Part model, mm, in its own coordinate system. Give positions to 0.01 mm unless a question says otherwise; leave off trailing zeros. Write each loop counter-clockwise with the first axis right and the second up, starting at its lowest first coordinate (ties: lowest second). Pieces come first, ordered by that corner, then holes.
from build123d import *

# Parameters (mm, degrees)
F1_DEPTH = 9.525


with BuildPart() as f1:
    # F0 (on Right) → F1 (new body)
    with BuildSketch(Plane.YZ):
        with BuildLine():
            Line((-686.6, 0), (-54.565425, 0))
            ThreePointArc((-54.565425, 0), (-17.701558, 16.22049), (-4.75569, 54.357787))
            Line((-4.75569, 54.357787), (-56.006549, 640.157787))
            ThreePointArc((-56.006549, 640.157787), (-72.036774, 672.663867), (-105.816284, 685.8))
            Line((-105.816284, 685.8), (-292.97298, 685.8))
            ThreePointArc((-292.97298, 685.8), (-312.355559, 681.890298), (-328.706935, 670.772624))
            Line((-328.706935, 670.772624), (-722.333955, 268.576607))
            ThreePointArc((-722.333955, 268.576607), (-732.896316, 252.489192), (-736.6, 233.603983))
            Line((-736.6, 233.603983), (-736.6, 50))
            ThreePointArc((-736.6, 50), (-721.955339, 14.644661), (-686.6, 0))
        make_face()
    extrude(amount=F1_DEPTH)


solid = f1.part
1) Mould opens along X. For faces 1 (the flat face through (9.525, -294, 272)), 2 (the cylindrical face through (4.696, -722.342, 15.036)), 3 (the flat face through (0, -294, 272)) say: +X half, -X half, draft (parallel to the pull), parting line (faces both ways), or undercut.
Check result:
face 1: +X half
face 2: draft
face 3: -X half
2) Saw through at C-C (z = 524). Write the cut outline in (x, y) (1 decimal).
Check result:
outline: (0, -472.4) - (9.5, -472.4) - (9.5, -45.8) - (0, -45.8) - close
3) Saw through at B-B (y = -474). Write the cut outline in (x, z) (3 decimals).
Check result:
outline: (0, 0) - (9.525, 0) - (9.525, 522.317) - (0, 522.317) - close
4) Drill centre lines: L1, parallel to Z at x = 5.5, y = -605.5; L2, parallel to Z at x = 9.25, y = -81; L3, parallel to Y at x = 6.5, z = 339. Where is each one in solid material? Low to high.
Check result:
L1: z = 0 to 387.95
L2: z = 0 to 679.21
L3: y = -653.41 to -29.66
5) Flat gauge pins, fed straight in: P1, Ø5, axis at x = 6, y = -545, coming from the +Z side; P2, Ø1, axis at x = 1.5, z = 293, coming from the -Y side; P3, Ø4, axis at x = 7.5, z = 73.5, coming from the +Y side. Where does each tip first touch, or does it go through?
Check result:
P1: stops at z = 452.33
P2: stops at y = -698.92
P3: stops at y = -6.26
6) Saw through at A-A (x = 3). Write the cut outline in (y, z), and give its area (3 significant figures).
Check result:
outline: (-736.6, 50) arc R50 ccw to (-686.6, 0) - (-54.57, 0) arc R50 ccw to (-4.76, 54.36) - (-56.01, 640.16) arc R50 ccw to (-105.82, 685.8) - (-292.97, 685.8) arc R50 ccw to (-328.71, 670.77) - (-722.33, 268.58) arc R50 ccw to (-736.6, 233.6) - close
area: 392,000 mm2
